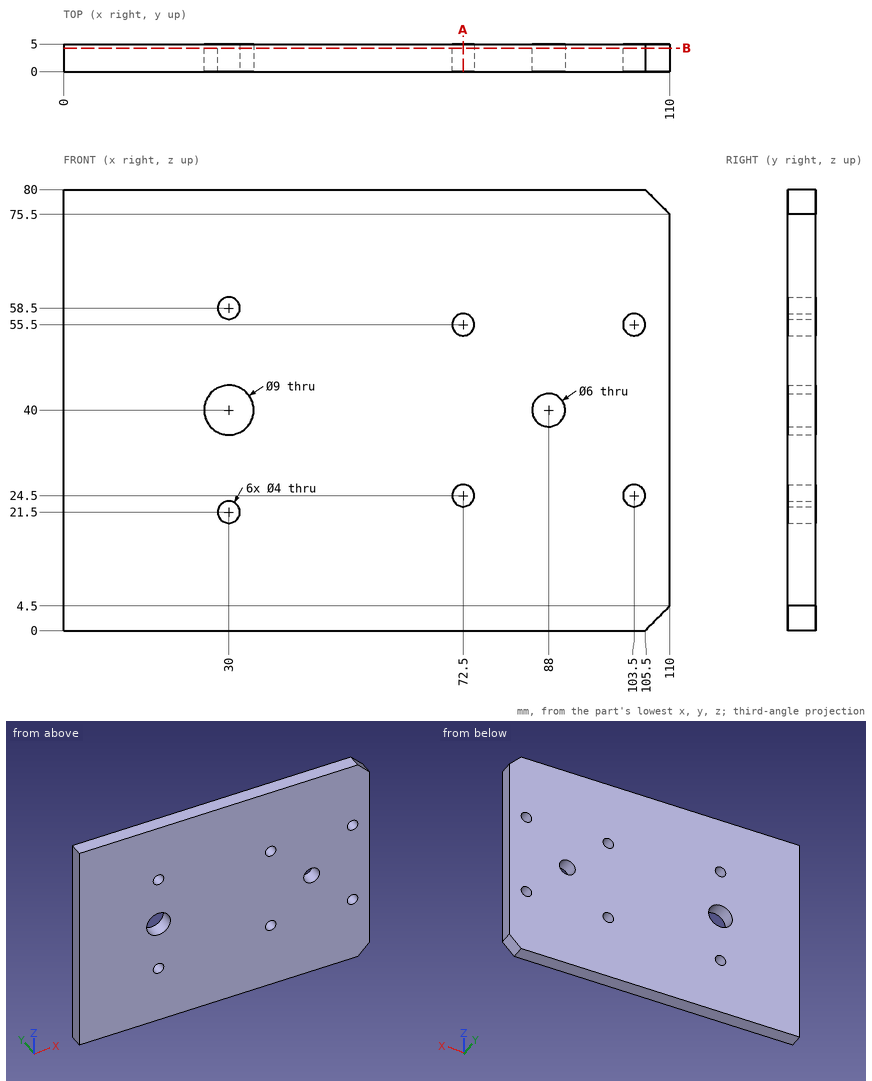
Here's the drawing with two shaded views (mm, measured from the low corner). I have some questions. Give positions to 0.01 mm unless a question says otherwise; leave off trailing zeros. Order: outer loops, then holes, each group sorted by start corner. A loop starts at its lowest first (then second) coordinate and runs counter-clockwise, first axis right, second up. Notation, with made-up numbers: (43, -37.5) -> (49, -37.5) arc R32 ccw to (49, -2.5) -> close; hole circle Ø9 at (20.5, 40). An arc over 180 degrees is marked (long way). One line per item, written item: value. Start each with the question number.
1. Imagine slicing it at B-B, the plane y = 4.25. Count the separate pieces of the cut face and the enclosed holes in it, plus the area to 3 significant figures.
2. Imagine slicing it at A-A, the plane x = 72.5. List the corners of the cut face in (y, z) for me, plus the area to 3 significant figures.
3. Will these pins go through, and if not, where does the flat tip stop? pin 1 Ø2.5 at (x, z) = (30, 21.5) entering from -Y; pin 2 Ø5 at (x, z) = (72.5, 24.5) entering from +Y.
4. I need wall thicknesses on probe 1 along Z at (x, y) = (72.5, 3.6); probe 2 along Z at (x, y) = (30, 1.9); probe 3 along Z at (x, y) = (27.5, 0.5). Which ranges of each line are inside material? Lowest first, please. Write a range as from..to.
Values follow:
1. separate pieces: 1
1. enclosed holes: 8
1. area: 8,610 mm2
2. outline: (0, 0) -> (5, 0) -> (5, 22.5) -> (0, 22.5) -> close; (0, 26.5) -> (5, 26.5) -> (5, 53.5) -> (0, 53.5) -> close; (0, 57.5) -> (5, 57.5) -> (5, 80) -> (0, 80) -> close
2. area: 360 mm2
3. pin 1: passes through
3. pin 2: stops at y = 5
4. probe 1: z = 0..22.5, 26.5..53.5, 57.5..80
4. probe 2: z = 0..19.5, 23.5..35.5, 44.5..56.5, 60.5..80
4. probe 3: z = 0..36.26, 43.74..80
